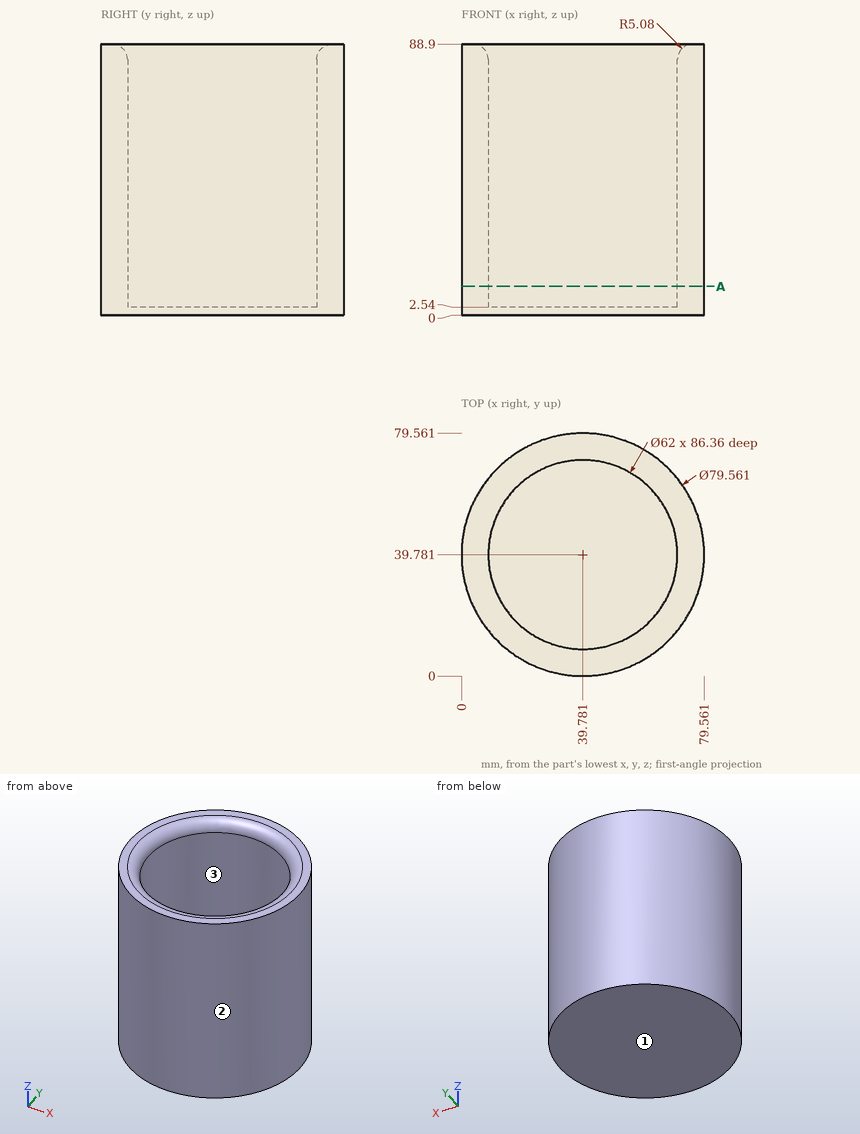
Can you work these out from the drawing? Everything is in mm from the part's minimum corner. Coordinates: 2 decimals unless noted, no trailing zeros. Order: outer loops, then holes, each group sorted by start corner. A loop starts at its lowest first (then second) coordinate and runs counter-clockwise, first axis right, second up. Notation, with made-up numbers: (74.5, 25.5) -> (93.5, 25.5) arc R19 cw to (93.5, 31.5) -> close; hole circle Ø5 at (-34, 39). An arc over 180 degrees is marked (long way). Return JSON: item names as keys, results as strings.
1) If I drill on probe 1 along X at (y, z) = (40.5, 16.5) (1 decimal); probe 2 along Y at (x, z) = (46.5, 21.5); probe 3 along X at (y, z) = (64, 49) (1 decimal), over which ranges is the centre line in solid material (lowest first)?
Conclusion:
{"probe 1": "x = 0 to 8.8, 70.8 to 79.6", "probe 2": "y = 0.57 to 9.52, 70.04 to 78.99", "probe 3": "x = 8.2 to 20.4, 59.1 to 71.3"}
2) If we section it at A-A on z = 9.5: List the corners of the cut face in (x, y) for me.
Conclusion:
{"outline": "circle Ø79.56 at (39.78, 39.78); hole circle Ø62 at (39.78, 39.78)"}
3) Thinking about a two-plate mould opening in X: for the marked faces 1, 2 and 3, which applies, +X half, -X half, draft (parallel to the pull), parting line (faces both ways), or undercut?
Conclusion:
{"face 1": "draft", "face 2": "parting line", "face 3": "undercut"}
4) I'm going to push flat-ended pins straight in: P1, Ø5, axis at y = 49.5, z = 25.5, coming from the +X side; P2, Ø1.5, axis at y = 53, z = 18.5, coming from the -X side (1 decimal); P3, Ø6, axis at y = 34, z = 48, coming from the -X side. Where does each tip first touch, or does it pass through?
Conclusion:
{"P1": "stops at x = 78.9", "P2": "stops at x = 2", "P3": "stops at x = 0.1"}
